Source: CAD feature listing. Evaluate the final solid. Frame: model axes, mm. Face numbers are marked on the shaded views. Give positions to 0.01 mm unless a question says otherwise; leave off trailing zeros. Loops run counter-clockwise (first coordinate to the right, second up) from the corner with the lowest first, then second, coordinate; pieces in that order, holes last. Notation, with made-up numbers: (47.5, -31.75) -> (92.5, -31.75) arc R28 ccw to (92.5, 4.25) -> close; hole circle Ø2 at (47, -32). An arc over 180 degrees is marked (long way). Return JSON: item names as keys, results as strings. Group by question number.
(1) Ray query, line 1 (Y direction, x = -15.5, z = 8); line 2 (X direction, y = -128, z = 4.5); line 3 (X direction, y = 113.6, z = 2.25). Return the intervals inside material, ascending. Write a range as from..to.
(2) Pin query (flat end, axial travel): pin 1 (12 mm diameter, centred on x = 74.71, y = -134.05, fed in from +Z); pin 2 (3 mm diameter, centred on x = 74, y = 75, fed in from +Z) (3 decimals). Return the tip coordinate at first contact, or that it passes through.
(3) Draft query along Y for the marked faces 1 and 2. Return one class per face: released by +Y, released by -Y, zero draft, split by the parting line, or undercut.
(4) Cut plane A-A on y = 58. Return loops of the section in (x, z) (1 decimal).
(5) Cut plane B-B on x = -11. Return loops of the section in (y, z) (3 decimals), then the cut area to 3 significant figures.
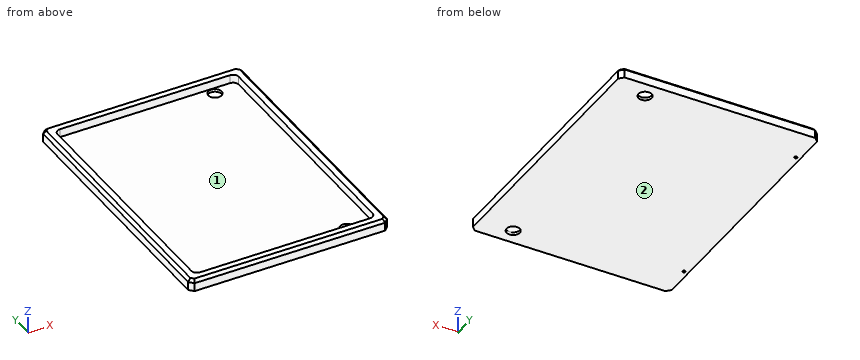
```python
from build123d import *

# Parameters (mm, degrees)
SKETCH1_W                 = 225.425
SKETCH1_H                 = 304.8
BOSS_EXTRUDE1_DEPTH       = 12.7
CUT_EXTRUDE1_DEPTH        = 9.525
SKETCH4_R                 = 7.5
CUT_EXTRUDE3_DEPTH        = 13.7
M4X0_7_TAPPED_HOLE1_D     = 3.3
M4X0_7_TAPPED_HOLE1_DEPTH = 8
M4X0_7_TAPPED_HOLE1_TIP   = 0.991420021
CHAMFER1_SIZE             = 4.7625
CHAMFER2_SIZE             = 3.175


with BuildPart() as part:
    # Sketch1 → Boss-Extrude1 (new body)
    with BuildSketch(Plane.XY):
        Rectangle(SKETCH1_W, SKETCH1_H)
    extrude(amount=BOSS_EXTRUDE1_DEPTH)

    # Sketch2 → Cut-Extrude1 (cut)
    with BuildSketch(Plane.XY.offset(12.7)):
        with BuildLine():
            Line((96.3625, -142.4), (-96.3625, -142.4))
            ThreePointArc((-96.3625, -142.4), (-100.852628061, -140.540128061), (-102.7125, -136.05))
            Line((-102.7125, -136.05), (-102.7125, 136.05))
            ThreePointArc((-102.7125, 136.05), (-100.852628061, 140.540128061), (-96.3625, 142.4))
            Line((-96.3625, 142.4), (96.3625, 142.4))
            ThreePointArc((96.3625, 142.4), (100.852628061, 140.540128061), (102.7125, 136.05))
            Line((102.7125, 136.05), (102.7125, -136.05))
            ThreePointArc((102.7125, -136.05), (100.852628061, -140.540128061), (96.3625, -142.4))
        make_face()
    extrude(amount=-CUT_EXTRUDE1_DEPTH, mode=Mode.SUBTRACT)

    # Sketch4 → Cut-Extrude3 (cut, through all)
    with BuildSketch(Plane(origin=(0, 0, 0), x_dir=(-1, 0, 0), z_dir=(0, 0, -1))):
        with Locations((-74.7125, -134.05)):
            Circle(SKETCH4_R)
        with Locations((-74.7125, 134.05)):
            Circle(SKETCH4_R)
    extrude(amount=-CUT_EXTRUDE3_DEPTH, mode=Mode.SUBTRACT)

    # M4x0.7 Tapped Hole1
    with Locations(Plane(origin=(0, 0, 0), x_dir=(-1, 0, 0), z_dir=(0, 0, -1))):
        with Locations((107.7125, -113.6), (107.7125, 113.6)):
            Hole(M4X0_7_TAPPED_HOLE1_D / 2, depth=M4X0_7_TAPPED_HOLE1_DEPTH)
            with Locations((0, 0, -(M4X0_7_TAPPED_HOLE1_DEPTH + M4X0_7_TAPPED_HOLE1_TIP / 2))):  # 118° drill point
                Cone(0, M4X0_7_TAPPED_HOLE1_D / 2, M4X0_7_TAPPED_HOLE1_TIP, mode=Mode.SUBTRACT)

    # Chamfer1
    chamfer1_edges = [part.edges().sort_by_distance(p)[0] for p in [
        (-112.7125, 152.4, 6.35),
        (112.7125, 152.4, 6.35),
        (112.7125, -152.4, 6.35),
        (-112.7125, -152.4, 6.35),
    ]]
    chamfer(chamfer1_edges, length=CHAMFER1_SIZE)

    # Chamfer2
    chamfer2_edges = [part.edges().sort_by_distance(p)[0] for p in [
        (-112.7125, 0, 12.7),
        (0, 152.4, 12.7),
        (0, -152.4, 12.7),
        (112.7125, 0, 12.7),
        (-110.33125, -150.01875, 12.7),
        (110.33125, -150.01875, 12.7),
        (110.33125, 150.01875, 12.7),
        (-110.33125, 150.01875, 12.7),
    ]]
    chamfer(chamfer2_edges, length=CHAMFER2_SIZE)


solid = part.part
```
Answers:
{
 "1": {"line 1": "-152.4..-142.4, 142.4..152.4", "line 2": "-112.71..-102.71, 102.71..112.71", "line 3": "-112.71..-109.36, -106.06..112.71"},
 "2": {"pin 1": "through", "pin 2": "z = 3.175"},
 "3": {"face 1": "undercut", "face 2": "zero draft"},
 "4": {"outline": "(-112.7, 0) -> (112.7, 0) -> (112.7, 9.5) -> (109.5, 12.7) -> (102.7, 12.7) -> (102.7, 3.2) -> (-102.7, 3.2) -> (-102.7, 12.7) -> (-109.5, 12.7) -> (-112.7, 9.5) -> close"},
 "5": {"outline": "(-152.4, 0) -> (152.4, 0) -> (152.4, 9.525) -> (149.225, 12.7) -> (142.4, 12.7) -> (142.4, 3.175) -> (-142.4, 3.175) -> (-142.4, 12.7) -> (-149.225, 12.7) -> (-152.4, 9.525) -> close", "area": "1,150 mm²"}
}
